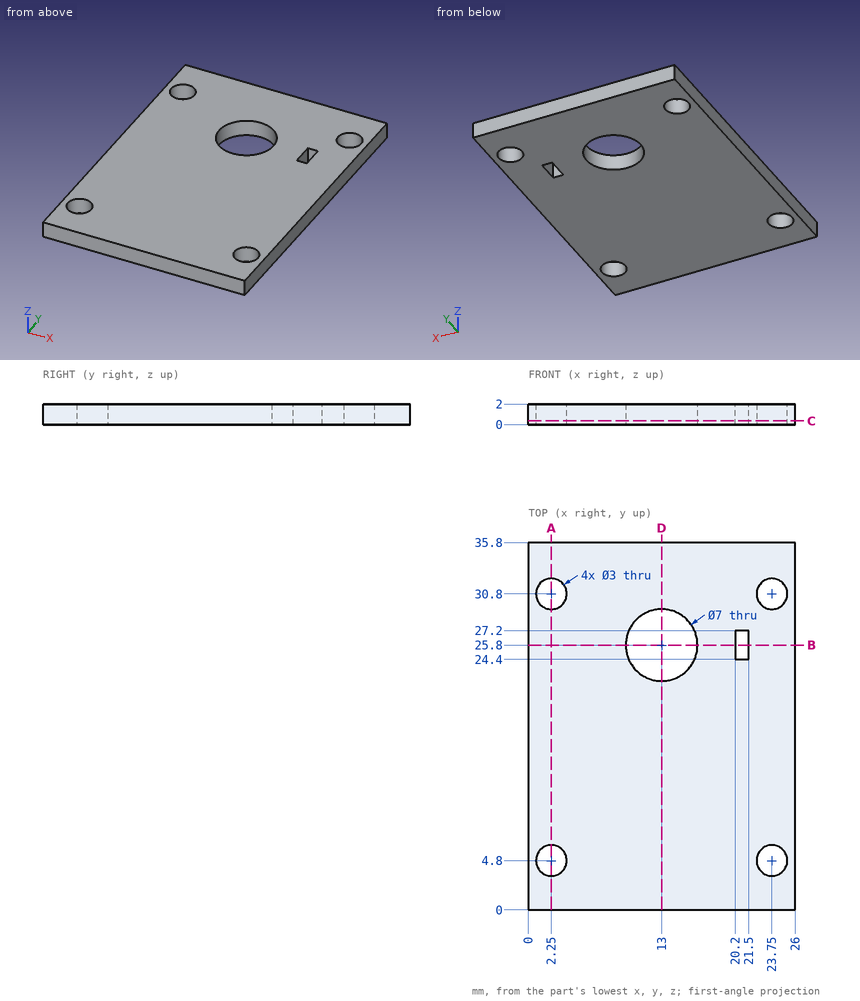
Source: three-view drawing plus pictorial views. Frame: mm from the lowest corner of the part. Give positions to 0.01 mm unless a question says otherwise; leave off trailing zeros. Order: outer loops, then holes, each group sorted by start corner. A loop starts at its lowest first (then second) coordinate and runs counter-clockwise, first axis right, second up. Notation, with made-up numbers: M 21.25,24 L 43.25,24 A26 ccw 43.25,54 Z; hole C 13.5,-21 d6. An arc over 180 degrees is marked long. One line per question, with ' | ' between items. Start each with the question number.
1. Section query B-B (y = 25.8). Return the cut outline in (x, z), and give its area (3 significant figures).
2. Material intervals for probe 1 along Y at (x, z) = (23.75, 0.6); probe 2 along X at (y, z) = (3.5, 1.4); probe 3 along Y at (x, z) = (13, 1.15), sorted ascending. Write a range as [from, to].
3. Section query C-C (z = 0.35). Return the cut outline in (x, y), and give its area (3 significant figures).
4. Section query D-D (x = 13). Return the cut outline in (y, z), and give its area (3 significant figures).
5. First-contact query: pin 1 Ø2.5 at (x, y) = (2.25, 30.8) entering from +Z. Flat tip, straight axial feed; report the tip coordinate or a pass-through.
6. Section query A-A (x = 2.25). Return the cut outline in (y, z), and give its area (3 significant figures).
Here are the results:
1) outline: M 0,0 L 9.5,0 L 9.5,2 L 0,2 Z; M 16.5,0 L 20.2,0 L 20.2,2 L 16.5,2 Z; M 21.5,0 L 26,0 L 26,2 L 21.5,2 Z | area: 35.4 mm²
2) probe 1: [0, 3.3], [6.3, 29.3], [32.3, 35.8] | probe 2: [0, 1.5], [3, 23], [24.5, 26] | probe 3: [0, 22.3], [29.3, 35.8]
3) outline: M 0,0 L 26,0 L 26,35.8 L 0,35.8 Z; hole C 2.25,4.8 d3; hole C 2.25,30.8 d3; hole C 13,25.8 d7; hole M 20.2,24.4 L 21.5,24.4 L 21.5,27.2 L 20.2,27.2 Z; hole C 23.75,4.8 d3; hole C 23.75,30.8 d3 | area: 860 mm²
4) outline: M 0,0 L 22.3,0 L 22.3,2 L 0,2 Z; M 29.3,0 L 35.8,0 L 35.8,2 L 29.3,2 Z | area: 57.6 mm²
5) pin 1: through
6) outline: M 0,0 L 3.3,0 L 3.3,2 L 0,2 Z; M 6.3,0 L 29.3,0 L 29.3,2 L 6.3,2 Z; M 32.3,0 L 35.8,0 L 35.8,2 L 32.3,2 Z | area: 59.6 mm²
